Autodesk Inventor part; units mm, degrees
ref_plane "YZ Plane" through (0, 0, 0) normal (1, 0, 0) x (0, 1, 0)
ref_plane "XZ Plane" through (0, 0, 0) normal (0, 1, 0) x (-1, 0, 0)
ref_plane "XY Plane" through (0, 0, 0) normal (0, 0, 1) x (1, 0, 0)
sketch "Sketch1" plane through (0, 0, 0) normal (0, 1, 0) x (-1, 0, 0)
  line L0 (0, 0) -> (100, 0)
  line L1 (100, 0) -> (100, -100)
  line L2 (100, -100) -> (0, -100)
  line L3 (0, -100) -> (0, 0)
  dimension "d0" = 100
  dimension "d1" = 100
  dimension "d2" = 100
extrude "Extrusion1" add sketch "Sketch1" along normal blind 20
sketch "Sketch2" plane through (0, 20, 0) normal (0, 1, 0) x (1, 0, 0)
  line L0 (-100, 100) -> (-100, 0)
  line L1 (0, 100) -> (-100, 100)
  line L2 (-100, 0) -> (0, 0)
  circle A0 centre (-50, 50) radius 25
  dimension "d5" = 50
extrude "Extrusion2" add sketch "Sketch2" along normal blind 150
sketch "Sketch3" plane through (-50, 170, -50) normal (0, 1, 0) x (1, 0, 0)
  circle A0 centre (0, 0) radius 25
  line L0 (0, 25) -> (35, 25)
  line L1 (35, 25) -> (35, -25)
  line L2 (0, 25) -> (-35, 25)
  line L3 (-35, 25) -> (-35, -25)
  line L4 (-35, -25) -> (35, -25)
  point P0 (50, -50)
  dimension "d12" = 35
  dimension "d13" = 35
extrude "Extrusion3" add sketch "Sketch3" along normal blind 20
sketch "Sketch4" plane through (-50, 190, -50) normal (0, 1, 0) x (1, 0, 0)
  line L0 (0, 25) -> (-35, 25)
  line L1 (-35, 25) -> (-25, 25)
  line L2 (-25, 25) -> (-25, -25)
  line L3 (-35, -25) -> (0, -25)
  line L4 (-35, -25) -> (-35, 25)
  line L5 (35, 25) -> (0, 25)
  line L6 (35, 25) -> (25, 25)
  line L7 (25, 25) -> (25, -25)
  line L8 (0, -25) -> (35, -25)
  line L9 (35, -25) -> (35, 25)
  point P0 (50, -50)
  dimension "d14" = 10
  dimension "d15" = 10
extrude "Extrusion4" add sketch "Sketch4" along normal blind 90 contours L2 L3 L4 L0 | L5 L9 L8 L7
sketch "Sketch5" plane through (-75, 190, -25) normal (1, 0, 0) x (0, 0, -1)
  line L0 (50, 0) -> (50, 90)
  line L1 (0, -20) -> (0, 90)
  circle A0 centre (25, 70) radius 10
  line L2 (50, 90) -> (0, 90)
  point P0 (-25, -190)
  dimension "d20" = 20
sketch "Sketch6" plane through (-15, 170, -25) normal (1, 0, 0) x (0, 0, -1)
  line L0 (50, 20) -> (50, 110)
  line L1 (50, 110) -> (50, 70)
  circle A0 centre (25, 90) radius 10
  line L2 (0, 110) -> (50, 110)
  point P0 (-25, -170)
  dimension "d23" = 20
extrude "Extrusion5" cut sketch "Sketch6" against normal blind 10
extrude "Extrusion6" cut sketch "Sketch5" against normal blind 10
fillet "Fillet1" radius 5 2 edges at (-25, 190, -50) (-75, 190, -50)
fillet "Fillet2" radius 10 4 edges at (-20, 280, -25) (-20, 280, -75) (-80, 280, -75) (-80, 280, -25)
fillet "Fillet3" radius 10 1 edges at (-75, 20, -50)
properties part number "wheel connector" material "Stainless Steel"
Design review of the part built by this model. Coordinates are the model's own, in mm. A direction names the side the tool comes from. Round coordinates to 2 decimals unless told otherwise and drop trailing zeros. Order: outer loops, then holes, each group sorted by start corner. A loop starts at its lowest first (then second) coordinate and runs counter-clockwise, first axis right, second up.
1) Consider section B-B (z = -50). State the section outline as (x, y) points.
The answers:
outline: (-100, 0) - (0, 0) - (0, 20) - (-15, 20) arc R10 cw to (-25, 30) - (-25, 170) - (-15, 170) - (-15, 250) - (-25, 250) - (-25, 195) arc R5 cw to (-30, 190) - (-70, 190) arc R5 cw to (-75, 195) - (-75, 250) - (-85, 250) - (-85, 170) - (-75, 170) - (-75, 30) arc R10 cw to (-85, 20) - (-100, 20) - close; (-85, 270) - (-75, 270) - (-75, 280) - (-85, 280) - close; (-25, 270) - (-15, 270) - (-15, 280) - (-25, 280) - close
2) Draft analysis for pull direction X (two halves, no side actions). For faces 1 (the flat face through (-20, 280, -50)), 2 (the cylindrical face through (-27, 191, -50)), 3 (the flat face through (-15, 224, -50)), state which applies: released by +X, released by -X, zero draft, split by the parting line, or undercut.
The answers:
face 1: zero draft
face 2: undercut
face 3: released by +X
3) Clearance check with flat-ended pins moving along their axes: pin 1 Ø23 at (y, z) = (260, -50) entering from -X; pin 2 Ø15 at (y, z) = (257, -45) entering from +X; pin 3 Ø12 at (x, y) = (-31.5, 139.5) entering from +Z; pin 4 Ø17.5 at (x, z) = (-33, -56) entering from -Y. State where each tip first meets the part, or that it passes through.
The answers:
pin 1: stops at x = -85
pin 2: stops at x = -15
pin 3: stops at z = -28.35
pin 4: stops at y = 0
4) Consider section D-D (z = -94). State the section outline as (x, y) points.
The answers:
outline: (-100, 0) - (0, 0) - (0, 20) - (-100, 20) - close
5) Consider section A-A (y = 260). State the section outline as (x, z) points.
The answers:
outline: (-85, -75) - (-75, -75) - (-75, -60) - (-85, -60) - close; (-85, -40) - (-75, -40) - (-75, -25) - (-85, -25) - close; (-25, -75) - (-15, -75) - (-15, -60) - (-25, -60) - close; (-25, -40) - (-15, -40) - (-15, -25) - (-25, -25) - close
6) For L1, parallel to Y at x = -19.5, z = -50; L2, parallel to Y at x = -21, z = -50; L3, parallel to X at y = 263, z = -32, list the stretches that pass through material, from the lowest coordinate up.
The answers:
L1: y = 0 to 21.07, 170 to 250, 270 to 280
L2: y = 0 to 22, 170 to 250, 270 to 280
L3: x = -85 to -75, -25 to -15
7) Consider section C-C (x = -21). Count the separate pieces of the cut face and the enclosed holes in it, plus the area to 3 significant figures.
The answers:
separate pieces: 2
enclosed holes: 1
area: 7,180 mm2
8) Machinability: for faces 4 (the flat face through (-50, 186, -25)), 5 (the flat face through (-25, 237, -50)), 6 (the flat face through (-85, 224, -50)), which of the approach directions +Z, -Z, +X, -X, +Y, -Y give a long, thin tool a straight path to every point of the face, cutting with its end or side? Answer none if there is none.
The answers:
face 4: +Z, +X, -X, +Y
face 5: +Z, -Z, +Y
face 6: +Z, -Z, -X, +Y
